from build123d import *

# Parameters (mm, degrees)
F4_R     = 12.5
F0_DEPTH = 55
F1_W     = 25
F1_H     = 25
F5_DEPTH = 55
F2_D     = 12
F7_R     = 10.5
F3_DEPTH = 50


with BuildPart() as f0:
    # F4 (on Top) → F0 (new body)
    with BuildSketch(Plane.XY):
        Circle(F4_R)
    extrude(amount=F0_DEPTH)

    # F1 (on Top) → F5 (join)
    with BuildSketch(Plane.XY):
        with Locations((-0.028275, -12.5)):
            Rectangle(F1_W, F1_H)
    extrude(amount=F5_DEPTH)

    # F2 (through all)
    with Locations(Plane(origin=(0, 0, 0), x_dir=(1, 0, 0), z_dir=(0, 0, -1))):
        with Locations((0, 0)):
            Hole(F2_D / 2)

    # F7 (on Top) → F3 (cut)
    with BuildSketch(Plane.XY):
        Circle(F7_R)
    extrude(amount=F3_DEPTH, mode=Mode.SUBTRACT)


solid = f0.part
Build history of the part. All positions in model axes, mm. A direction names the side the tool comes from. Round coordinates to 2 decimals unless told otherwise and drop trailing zeros. Loops run counter-clockwise (first coordinate to the right, second up) from the corner with the lowest first, then second, coordinate; pieces in that order, holes last. Notation, with made-up numbers: (72.5, 52.5) -> (116.5, 52.5) arc R6 cw to (116.5, 62.5) -> close; hole circle Ø11 at (-37, 36). An arc over 180 degrees is marked (long way). Use CSV: the item, a comma, the result in double quotes. Start each with the question number.
Q1. Drill centre lines: L1, parallel to X at y = -0.5, z = 18.5; L2, parallel to Y at x = 0, z = 52.35; L3, parallel to Z at x = -5.75, y = 4.5. Where is each one in solid material? Low to high.
Q2. Which spindle directions (+Z, -Z, +X, -X, +Y, -Y) get a long thin tool onto all of the face, cutting with end or side? Do faces 1 (the face through (10, 3.2, 24.6)), 2 (the face through (6, 0, 53)). Say none if no direction does.
Q3. Saw through at C-C on y = -3.5. Give the cut face in (x, z).
Q4. Saw through at D-D on x = -7.5. Give the cut face in (y, z).
Q5. Mould opens along X. For faces 3 (the face through (12.472, -13, 27)), 4 (the face through (5, -5, 50)), 5 (the face through (0, -25, 27)), 6 (the face through (0.7, 12.48, 27.12)) say: +X half, -X half, draft (parallel to the pull), parting line (faces both ways), or undercut.
Q6. Saw through at A-A on x = 0. Give the cut face in (y, z), and give its area (4 significant figures).
Q7. Flat gauge pins, fed straight in: pin 1 Ø1.5 at (x, z) = (4.5, 12) entering from +Y; pin 2 Ø1.5 at (x, z) = (2, 24) entering from +Y; pin 3 Ø12 at (y, z) = (-17.5, 39.5) entering from +X; pin 4 Ø12 at (x, y) = (1, 1.5) entering from +Z. Where does each tip first touch, or does it go through?
Solutions:
1,L1,"x = -12.53 to -10.49, 10.49 to 12.49"
1,L2,"y = -25 to -6, 6 to 12.5"
1,L3,"z = 50 to 55"
2,face 1,"-Z"
2,face 2,"+Z, -Z"
3,outline,"(-12.53, 0) -> (-9.9, 0) -> (-9.9, 50) -> (-4.87, 50) -> (-4.87, 55) -> (-12.53, 55) -> close; (4.87, 50) -> (9.9, 50) -> (9.9, 0) -> (12.47, 0) -> (12.47, 55) -> (4.87, 55) -> close"
4,outline,"(-25, 0) -> (-7.35, 0) -> (-7.35, 50) -> (7.35, 50) -> (7.35, 0) -> (10, 0) -> (10, 55) -> (-25, 55) -> close"
5,face 3,"+X half"
5,face 4,"undercut"
5,face 5,"draft"
5,face 6,"parting line"
6,outline,"(-25, 0) -> (-10.5, 0) -> (-10.5, 50) -> (-6, 50) -> (-6, 55) -> (-25, 55) -> close; (6, 50) -> (10.5, 50) -> (10.5, 0) -> (12.5, 0) -> (12.5, 55) -> (6, 55) -> close"
6,area,"952.5 mm^2"
7,pin 1,"stops at y = 11.92"
7,pin 2,"stops at y = 12.44"
7,pin 3,"stops at x = 12.47"
7,pin 4,"stops at z = 55"
